Autodesk Inventor part; units mm, degrees
ref_plane "YZ Plane" through (0, 0, 0) normal (1, 0, 0) x (0, 1, 0)
ref_plane "XZ Plane" through (0, 0, 0) normal (0, 1, 0) x (-1, 0, 0)
ref_plane "XY Plane" through (0, 0, 0) normal (0, 0, 1) x (1, 0, 0)
sketch "Sketch1" plane through (0, 0, 0) normal (0, 0, 1) x (1, 0, 0)
  line L0 (0, 0) -> (-170.9112, 0)
  line L1 (-170.9112, 0) -> (-170.9112, -1500)
  line L2 (-170.9112, -1500) -> (0, -1500)
  line L3 (0, -1500) -> (0, 0)
  line L4 (-170.9112, -1400) -> (-81, -1400)
  line L5 (-81, -1400) -> (-81, -1394)
  line L6 (-81, -1394) -> (-170.9112, -1394)
  line L7 (-170.9112, -1394) -> (-170.9112, -1400)
  line L8 (-170.9112, -900) -> (-81, -900)
  line L9 (-81, -900) -> (-81, -894)
  line L10 (-81, -894) -> (-170.9112, -894)
  line L11 (-170.9112, -894) -> (-170.9112, -900)
  line L12 (-170.9112, -400) -> (-81, -400)
  line L13 (-81, -400) -> (-81, -394)
  line L14 (-81, -394) -> (-170.9112, -394)
  line L15 (-170.9112, -394) -> (-170.9112, -400)
  point P0 (-170.9112, -400)
  dimension "d0" = 1500
  dimension "d1" = 170.9112
  dimension "d2" = 6
  dimension "d4" = 100
  dimension "d7" = 500
  dimension "d23" = 81
extrude "Plate1" add sketch "Sketch1" along normal blind 4 contours L3 L2 L1 L4 L5 L6 L8 L9 L10 L12 L13 L14 L0
sketch "Sketch2" plane through (4, 0, 0) normal (-1, 0, 0) x (0, -1, 0)
  line L0 (1500, 0) -> (0, 0)
  line L1 (0, 0) -> (0, 35)
  line L2 (0, 35) -> (1500, 35)
  line L3 (1500, 35) -> (1500, 0)
edge flange "Flange1" height 35 angle 90 thickness 4 bend radius 4 thickness toward (-1, 0, 0) relief tear relief width 4 relief depth 2 edges at (0, -750, 4) wall of the first edge with corners at (4, -1500, 0) (4, 0, 0) (4, 0, 35) (4, -1500, 35)
bend "Bend1"
corner "Corner1"
equation "\"d1\" = Stringer3_deep"
equation "\"d12\" = Thickness"
equation "\"d13\" = BendReliefWidth"
equation "\"d14\" = BendReliefDepth"
equation "\"d15\" = MinimumRemnant"
equation "\"d16\" = TransitionRadius"
equation "\"d19\" = BendRadius"
equation "\"d20\" = CornerReliefSize"
equation "\"d21\" = GapSize"
equation "\"d22\" = JacobiRadiusSize"
equation "\"BendRadius\" = Thickness"
equation "\"BendReliefWidth\" = Thickness"
equation "\"BendReliefDepth\" = 0.5 * Thickness"
equation "\"CornerReliefSize\" = 4 * Thickness"
equation "\"MinimumRemnant\" = 2 * Thickness"
equation "\"TransitionRadius\" = BendRadius"
equation "\"JacobiRadiusSize\" = BendRadius"
equation "\"GapSize\" = Thickness"
properties part number "stringer 1.3" material "Steel"
Model file for the job. Use its own axes, mm. A direction names the side the tool comes from. Coordinates: 2 decimals unless noted, no trailing zeros. Order: outer loops, then holes, each group sorted by start corner. A loop starts at its lowest first (then second) coordinate and runs counter-clockwise, first axis right, second up. Notation, with made-up numbers: (28, 66) - (85, 66) arc R27 ccw to (85, 94) - close; hole circle Ø10 at (81.25, 53). An arc over 180 degrees is marked (long way). Return JSON: item names as keys, results as strings. Group by question number.
1) Saw through at B-B, the plane y = -650. Write the cut outline in (x, z).
2) Saw through at C-C, the plane z = 16. Write the cut outline in (x, y).
3) Tool access for faces 1 (the flat face through (0, -740, 21)), 2 (the flat face through (-64, 0, 3)): list every direction of +Z, -Z, +X, -X, +Y, -Y with a clear straight run to the whole face (end or side of a thin tool).
4) Saw through at A-A, the plane x = -123.5. Write the cut outline in (y, z), plus the area to 3 significant figures.
5) Flat gauge pins, fed straight in: P1, Ø4, axis at x = -90.5, y = -651.5, coming from the +Z side; P2, Ø4.5, axis at y = -897.5, z = 1.5, coming from the -X side; P3, Ø6, axis at y = -1058.5, z = 4.5, coming from the +X side. Where does each tip first touch, or does it go through?
6) Saw through at D-D, the plane x = -21.5. Write the cut outline in (y, z).
7) Probe line 1 (Y direction, x = -99.5, z = 2.5); line 2 (X direction, y = -119.5, z = 19.5); line 3 (X direction, y = -773, z = 7). List the from-to ranges inside material, lowest first. Write a range as from..to.
Values found:
{
 "1": {"outline": "(-170.91, 0) - (-4, 0) arc R8 ccw to (4, 8) - (4, 35) - (0, 35) - (0, 8) arc R4 cw to (-4, 4) - (-170.91, 4) - close"},
 "2": {"outline": "(0, -1500) - (4, -1500) - (4, 0) - (0, 0) - close"},
 "3": {"face 1": "+Z, -X, +Y, -Y", "face 2": "+Z, -Z, +X, -X, +Y"},
 "4": {"outline": "(-1500, 0) - (-1400, 0) - (-1400, 4) - (-1500, 4) - close; (-1394, 0) - (-900, 0) - (-900, 4) - (-1394, 4) - close; (-894, 0) - (-400, 0) - (-400, 4) - (-894, 4) - close; (-394, 0) - (0, 0) - (0, 4) - (-394, 4) - close", "area": "5,930 mm²"},
 "5": {"P1": "stops at z = 4", "P2": "stops at x = -81", "P3": "stops at x = 3.98"},
 "6": {"outline": "(-1500, 0) - (0, 0) - (0, 4) - (-1500, 4) - close"},
 "7": {"line 1": "y = -1500..-1400, -1394..-900, -894..-400, -394..0", "line 2": "x = 0..4", "line 3": "x = -0.13..3.94"}
}
